Job drawing, mm, ordinate dimensions from the low corner. One solid piece. Round coordinates to 2 decimals unless told otherwise and drop trailing zeros. Loops run counter-clockwise (first coordinate to the right, second up) from the corner with the lowest first, then second, coordinate; pieces in that order, holes last. Notation, with made-up numbers: M 36,1 L 94,1 A22 cw 94,8 Z; hole C -33,0.5 d3. An arc over 180 degrees is marked long. Put each result on its own line as item: value. Start each with the question number.
1) Slice it at B-B on x = 2.75. Give the cut face in (y, z).
2) Slice it at C-C on y = 1. Give the cut face in (x, z), then the cut area to 3 significant figures.
3) Slice it at A-A on x = 1.5. Give the cut face in (y, z).
4) Slice it at D-D on z = 6.5. Give the cut face in (x, y).
5) Probe line 1 along Z through (x, y) = (1.2, 5) (1 decimal); line 2 along Z through (x, y) = (2.55, 2.75) (1 decimal); line 3 along Y through (x, z) = (2.05, 4.5) (1 decimal). List the from-to ranges inside material, lowest first.
6) Pull direction Z, two halves, no side cores. Call the marked faces 1, 2 and 3: +Z half, -Z half, draft (parallel to the pull), parting line (faces both ways), or undercut.
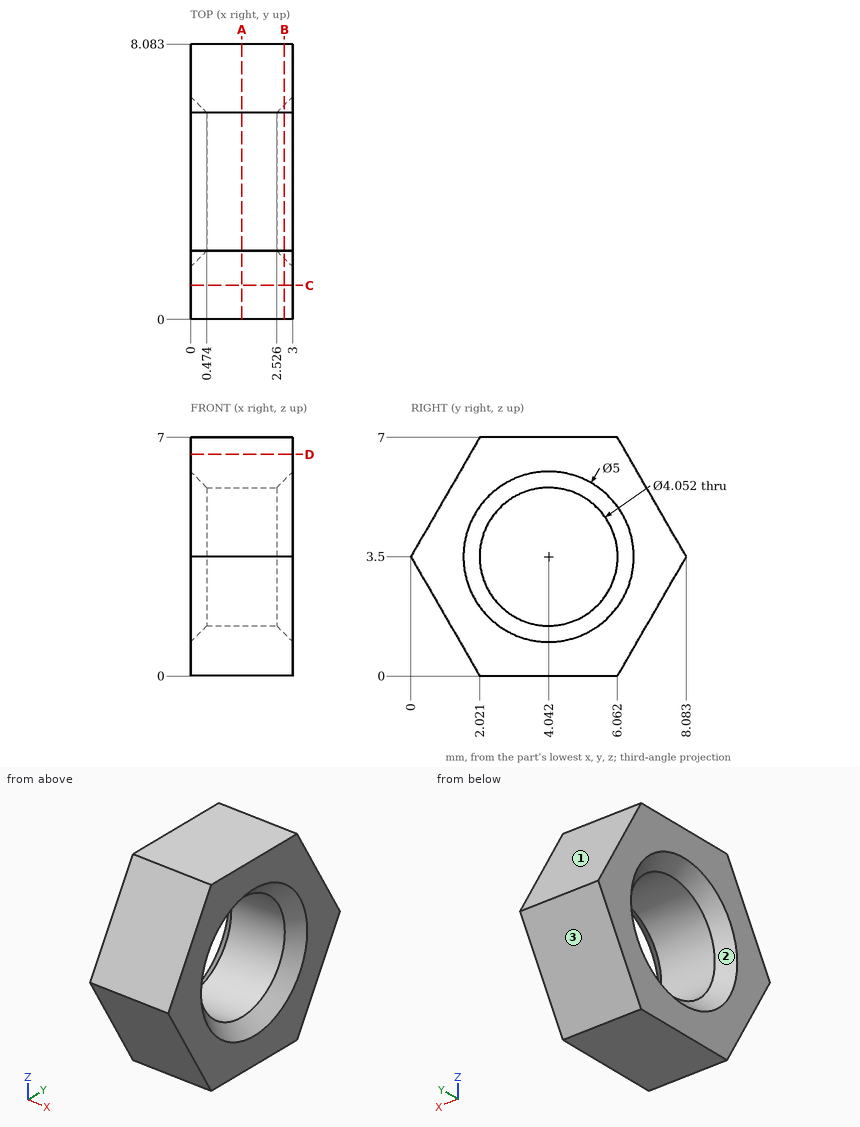
Recorded:
1. outline: M 0,3.5 L 2.02,0 L 6.06,0 L 8.08,3.5 L 6.06,7 L 2.02,7 Z; hole C 4.04,3.5 d4.5
2. outline: M 0,1.77 L 3,1.77 L 3,5.23 L 0,5.23 Z
2. area: 10.4 mm2
3. outline: M 0,3.5 L 2.02,0 L 6.06,0 L 8.08,3.5 L 6.06,7 L 2.02,7 Z; hole C 4.04,3.5 d4.05
4. outline: M 0,1.73 L 3,1.73 L 3,6.35 L 0,6.35 Z
5. line 1: z = 0 to 1.7, 5.3 to 7
5. line 2: z = 0 to 1.9, 5.1 to 7
5. line 3: y = 0.6 to 2.3, 5.8 to 7.5
6. face 1: +Z half
6. face 2: undercut
6. face 3: -Z half
